For this review, take the finished solid that the model builds, in its own axes (mm). A direction names the side the tool comes from. Round coordinates to 2 decimals unless told otherwise and drop trailing zeros. Loops run counter-clockwise (first coordinate to the right, second up) from the corner with the lowest first, then second, coordinate; pieces in that order, holes last. Notation, with made-up numbers: M -31.5,-3 L -0.5,-3 A29 ccw -0.5,36 Z; hole C 22.25,-27 d2. An arc over 180 degrees is marked long. Write item = value, one per line. Start each with the question number.
```python
from build123d import *

# Parameters (mm, degrees)
RESSALTO_EXTRUS_O1_DEPTH      = 263
RESSALTO_EXTRUS_O1_DEPTH_BACK = 92
LPATTERN1_COUNT               = 6
LPATTERN1_PITCH               = 40
LPATTERN1_COL_COUNT           = 4
LPATTERN1_COL_PITCH           = 40


with BuildPart() as part:
    # Esboço1 → Ressalto-extrusão1 (new, two sides: drawn at the far end of the back side and taken through both)
    with BuildSketch(Plane(origin=(-15, 0, 0), x_dir=(0, 0, -1), z_dir=(1, 0, 0)).offset(-RESSALTO_EXTRUS_O1_DEPTH_BACK)):
        with BuildLine():
            Line((-12, 4), (-12, 0.5))
            Line((-12, 0.5), (-11.5, 0))
            Line((-11.5, 0), (11.5, 0))
            Line((11.5, 0), (12, 0.5))
            Line((12, 0.5), (12, 4))
            Line((12, 4), (11.814562479, 5.051668439))
            ThreePointArc((11.814562479, 5.051668439), (10.518990309, 6.082939778), (11.383714346, 7.495129625))
            Line((11.383714346, 7.495129625), (11.206528587, 8.5))
            Line((11.206528587, 8.5), (-11.206528587, 8.5))
            Line((-11.206528587, 8.5), (-11.383714346, 7.495129625))
            ThreePointArc((-11.383714346, 7.495129625), (-10.518990309, 6.082939778), (-11.814562479, 5.051668439))
            Line((-11.814562479, 5.051668439), (-12, 4))
        make_face()
    extrude(amount=RESSALTO_EXTRUS_O1_DEPTH + RESSALTO_EXTRUS_O1_DEPTH_BACK)

    # Esboço3 → Corte-Revolução2 (revolve, cut)
    with BuildSketch(Plane.XY, mode=Mode.PRIVATE) as corte_revolu_o2_sk:
        Polygon((40, 8.5), (44, 8.5), (44, 4), (42.25, 4), (42.25, 0), (40, 0), align=None)
    corte_revolu_o2 = revolve(corte_revolu_o2_sk.sketch.rotate(Axis((40, 0, 0), (0, 1, 0)), 270), axis=Axis((40, 0, 0), (0, 1, 0)), mode=Mode.SUBTRACT)

    # LPattern1: Corte-Revolução2 ×6
    with Locations(*[(i * LPATTERN1_PITCH, 0, 0) for i in range(1, LPATTERN1_COUNT)]):
        add(corte_revolu_o2, mode=Mode.SUBTRACT)

    # LPattern1 col: Corte-Revolução2 ×4
    with Locations(*[(-i * LPATTERN1_COL_PITCH, 0, 0) for i in range(1, LPATTERN1_COL_COUNT)]):
        add(corte_revolu_o2, mode=Mode.SUBTRACT)


solid = part.part
```
(1) Draft analysis for pull direction X (two halves, no side actions). For faces 3 (the flat face through (68, 0, 0)), 4 (the flat face through (38, 4, 2)), 5 (the flat face through (248, 4, 0)), state which applies: +X half, -X half, draft (parallel to the pull), parting line (faces both ways), or undercut.
(2) Add section A-A on x = 213. Write out the cut boundary in (y, z).
(3) For pin 1 Ø6.5 at (x, z) = (240, 0) entering from -Y; pin 2 Ø7 at (x, z) = (40, 0) entering from +Y, all flat-tipped, find the tip position at first contact; note any pin that passes through.
(4) Wall thickness on L1, parallel to Z at x = 0, y = 1.2; L2, parallel to Z at x = 240, y = 6; L3, parallel to Z at x = 27.5, y = 6: over which ranges is each line inside the solid? List them lowest first.
(5) Tool access review of faces 1 (the flat face through (68, 8.5, 0)), 2 (the cylindrical face through (-83.905, 6.219, -0.867)): name each direction out of +Z, -Z, +X, -X, +Y, -Y from which nothing blocks a thin tool from reaching the whole face with its end or side.
Answer sheet:
q1.face_3 = draft
q1.face_4 = undercut
q1.face_5 = +X half
q2.outline = M 0,-11.5 L 0.5,-12 L 4,-12 L 5.05,-11.81 A1.25 cw 7.5,-11.38 L 8.5,-11.21 L 8.5,11.21 L 7.5,11.38 A1.25 cw 5.05,11.81 L 4,12 L 0.5,12 L 0,11.5 Z
q3.pin_1 = 0
q3.pin_2 = 4
q4.L1 = -12 to -2.25, 2.25 to 12
q4.L2 = -10.54 to -4, 4 to 10.54
q4.L3 = -10.54 to 10.54
q5.face_1 = +Z, -Z, +X, -X, +Y
q5.face_2 = +Y
